Read the model definition and answer for the solid it produces. Units are mm, in the model's axes. A direction names the side the tool comes from. Round coordinates to 2 decimals unless told otherwise and drop trailing zeros. Write each loop counter-clockwise with the first axis right and the second up, starting at its lowest first coordinate (ties: lowest second). Pieces come first, ordered by that corner, then holes. Notation, with made-up numbers: (40.5, 87) - (44.5, 87) arc R20 cw to (44.5, 121) - close; hole circle Ø5 at (83, 60). An arc over 180 degrees is marked (long way). Answer as CSV lines item,"result". Start each with the question number.
1) Which of the six approach directions +Z, -Z, +X, -X, +Y, -Y give full straight-line access (tool end or side, diameter ignored) to faces 1 (the flat face through (-3.8, -5.7, 0)), 2 (the flat face through (9, 1, -14)), 3 (the flat face through (-3.8, 5.7, 0)), 4 (the flat face through (3.8, -5.6, 0)), 5 (the flat face through (3.8, 5.7, 0))?
2) Each of these flat-tipped pins is pushed along its axis until it touches: pin 1 (1.1 mm diameter, centred on x = 9, z = -13.5, fed in from +Y); pin 2 (1 mm diameter, centred on x = -3, z = 7.5, fed in from +Y); pin 3 (3.5 mm diameter, centred on y = 3, z = -5.5, fed in from +X). Where does it stop, or does it pass through?
3) Find section C-C on z = 1. Determine the outline of the cut face in (x, y), then the cut area to 3 significant figures.
4) Find section A-A on x = 4.25. Determine the outline of the cut face in (y, z).
5) Find section B-B on y = -1. Determine the outline of the cut face in (x, z), then the cut area to 3 significant figures.
6) Find section D-D on x = 6.75. Determine the outline of the cut face in (y, z).
7) Consider line 1 along X through (y, z) = (0.5, -12.5); line 2 along Z through (x, y) = (7.75, -1.25); line 3 along Z through (x, y) = (12, 0.5). Determine where each line is inside the solid, lowest interval first.
from build123d import *

# Parameters (mm, degrees)
SKETCH1_W           = 5
SKETCH1_H           = 10
BOSS_EXTRUDE1_DEPTH = 15.1
SKETCH2_W           = 10
SKETCH2_H           = 12
BOSS_EXTRUDE2_DEPTH = 18
BOSS_EXTRUDE3_DEPTH = 8


with BuildPart() as part:
    # Sketch1 → Boss-Extrude1 (new body)
    with BuildSketch(Plane.XY):
        with Locations((-2.5, 0)):
            Rectangle(SKETCH1_W, SKETCH1_H)
        with Locations((2.5, 0)):
            Rectangle(SKETCH1_W, SKETCH1_H)
        with BuildLine():
            Line((0, 6), (0, 5))
            Line((0, 5), (5, 5))
            ThreePointArc((5, 5), (2.549509757, 5.747548784), (0, 6))
        make_face()
        with BuildLine():
            Line((-5, 5), (0, 5))
            Line((0, 5), (0, 6))
            ThreePointArc((0, 6), (-2.549509757, 5.747548784), (-5, 5))
        make_face()
        with BuildLine():
            Line((0, -5), (0, -6))
            ThreePointArc((0, -6), (2.549509757, -5.747548784), (5, -5))
            Line((5, -5), (0, -5))
        make_face()
        with BuildLine():
            ThreePointArc((-5, -5), (-2.549509757, -5.747548784), (0, -6))
            Line((0, -6), (0, -5))
            Line((0, -5), (-5, -5))
        make_face()
    extrude(amount=BOSS_EXTRUDE1_DEPTH)

    # Sketch2 → Boss-Extrude2 (add)
    with BuildSketch(Plane.XY):
        Rectangle(SKETCH2_W, SKETCH2_H)
    extrude(amount=-BOSS_EXTRUDE2_DEPTH)

    # Sketch3 → Boss-Extrude3 (add)
    with BuildSketch(Plane(origin=(5, 0, 0), x_dir=(0, 0, -1), z_dir=(1, 0, 0))):
        with BuildLine():
            Line((14, -1.5), (14, 0))
            Line((14, 0), (14, 1))
            Line((14, 1), (12.881966011, 1))
            ThreePointArc((12.881966011, 1), (12.630693606, -0.612372436), (14, -1.5))
        make_face()
        with BuildLine():
            Line((14, 0), (15.5, 0))
            ThreePointArc((15.5, 0), (15.401258538, 0.535233135), (15.118033989, 1))
            Line((15.118033989, 1), (14, 1))
            Line((14, 1), (14, 0))
        make_face()
        with BuildLine():
            ThreePointArc((14, -1.5), (15.060660172, -1.060660172), (15.5, 0))
            Line((15.5, 0), (14, 0))
            Line((14, 0), (14, -1.5))
        make_face()
    extrude(amount=BOSS_EXTRUDE3_DEPTH)


solid = part.part
Check values:
1,face 1,"+Z, -X, -Y"
1,face 2,"+Z, -Z, +X, +Y"
1,face 3,"+Z, -X, +Y"
1,face 4,"+Z, +X, -Y"
1,face 5,"+Z, +X, +Y"
2,pin 1,"stops at y = 1"
2,pin 2,"stops at y = 5.76"
2,pin 3,"stops at x = 5"
3,outline,"(-5, -5) arc R13 ccw to (5, -5) - (5, 5) arc R13 ccw to (-5, 5) - close"
3,area,"113 mm^2"
4,outline,"(-6, -18) - (6, -18) - (6, 0) - (5.29, 0) - (5.29, 15.1) - (-5.29, 15.1) - (-5.29, 0) - (-6, 0) - close"
5,outline,"(-5, -18) - (5, -18) - (5, -15.12) - (13, -15.12) - (13, -12.88) - (5, -12.88) - (5, 15.1) - (-5, 15.1) - close"
5,area,"349 mm^2"
6,outline,"(1, -15.12) - (1, -12.88) arc R1.5 ccw (long way) to start"
7,line 1,"x = -5 to 5"
7,line 2,"z = -14.83 to -13.17"
7,line 3,"z = -15.41 to -12.59"
